The model under review builds one solid part; all positions refer to its coordinate system, in mm. A direction names the side the tool comes from. Coordinates: 2 decimals unless noted, no trailing zeros. Loops run counter-clockwise (first coordinate to the right, second up) from the corner with the lowest first, then second, coordinate; pieces in that order, holes last. Notation, with made-up numbers: (89, -35) - (126, -35) arc R15 ccw to (126, -13) - close; hole circle Ø7 at (-7.75, -11.5). An arc over 180 degrees is marked (long way). Use a Markdown table: item, result. Add a question column.
1) Clearance check with flat-ended pins moving along their axes: pin 1 (1 mm diameter, centred on y = 4, z = 9, fed in from +X); pin 2 (2.5 mm diameter, centred on x = -27.5, z = -22.5, fed in from +Y); pin 3 (3 mm diameter, centred on y = 4.5, z = 17.5, fed in from -X); pin 4 (0.5 mm diameter, centred on x = 27, y = 0.5, fed in from -Z). State where each tip first meets the part, or that it passes through.
2) For faces 4 (the flat face through (26, 1, 21)), 5 (the flat face through (0, 1, 23)), 6 (the flat face through (0, 1, -20)), list the 3-axis set-ups (+Z, -Z, +X, -X, +Y, -Y) from which the entire face can be reached by the end or side of a thin tool; tool diameter is ignored.
3) To check wall thickness, follow L1, parallel to X at y = 0.85, z = 3; L2, parallel to X at y = 0.35, z = 22.5. State the ranges of each line that lie inside material, in increasing order. Write a range as [from, to].
4) Add section C-C, the plane y = 1.7. Give the boundary of the cut face in (x, z).
5) Add section A-A, the plane z = 22.5. Give the boundary of the cut face in (x, y), and give its area (3 significant figures).
6) Add section B-B, the plane x = -27.5. Give the boundary of the cut face in (y, z).
7) Add section D-D, the plane z = -22.5. Give the boundary of the cut face in (x, y).
8) The part is to be moulded in two halves that separate along X. For faces 1 (the flat face through (-3, 2, -25)), 2 (the cylindrical face through (-26.013, 0.507, -22.695)), 3 (the flat face through (15, 1, 20)), say which applies: pulls with the +X half, pulls with the -X half, needs draft (parallel to the pull), parting line crosses it, or undercut.
```python
from build123d import *

# Parameters (mm, degrees)
SKETCH1_W           = 50
SKETCH1_H           = 50
BOSS_EXTRUDE2_DEPTH = 5
SKETCH2_W           = 40
SKETCH2_H           = 40
CUT_EXTRUDE1_DEPTH  = 3
SKETCH3_W           = 5
SKETCH3_H           = 5
BOSS_EXTRUDE3_DEPTH = 1
SKETCH4_R           = 1.5
CUT_EXTRUDE2_DEPTH  = 1
SKETCH6_W           = 10
SKETCH6_H           = 3
CUT_EXTRUDE3_DEPTH  = 10


with BuildPart() as part:
    # Sketch1 → Boss-Extrude2 (new body)
    with BuildSketch(Plane(origin=(0, 0, 0), x_dir=(1, 0, 0), z_dir=(0, 1, 0))):
        Rectangle(SKETCH1_W, SKETCH1_H)
    extrude(amount=BOSS_EXTRUDE2_DEPTH)

    # Sketch2 → Cut-Extrude1 (cut)
    with BuildSketch(Plane(origin=(0, 0, 0), x_dir=(-1, 0, 0), z_dir=(0, -1, 0))):
        Rectangle(SKETCH2_W, SKETCH2_H)
    extrude(amount=-CUT_EXTRUDE1_DEPTH, mode=Mode.SUBTRACT)

    # Sketch3 → Boss-Extrude3 (add)
    with BuildSketch(Plane(origin=(0, 0, 0), x_dir=(-1, 0, 0), z_dir=(0, -1, 0))):
        with Locations((27.5, 22.5)):
            Rectangle(SKETCH3_W, SKETCH3_H)
        with Locations((-27.5, -22.5)):
            Rectangle(SKETCH3_W, SKETCH3_H)
    extrude(amount=-BOSS_EXTRUDE3_DEPTH)

    # Sketch4 → Cut-Extrude2 (cut)
    with BuildSketch(Plane(origin=(0, 1, 0), x_dir=(1, 0, 0), z_dir=(0, 1, 0))):
        with Locations(Location((-27.5, 22.5, 0), (0, 0, 270))):  # turned: the seam where the file's is
            Circle(SKETCH4_R)
        with Locations(Location((27.5, -22.5, 0), (0, 0, 270))):  # turned: the seam where the file's is
            Circle(SKETCH4_R)
    extrude(amount=-CUT_EXTRUDE2_DEPTH, mode=Mode.SUBTRACT)

    # Sketch6 → Cut-Extrude3 (cut)
    with BuildSketch(Plane.XY.offset(25)):
        with Locations((5, 1.5)):
            Rectangle(SKETCH6_W, SKETCH6_H)
    extrude(amount=-CUT_EXTRUDE3_DEPTH, mode=Mode.SUBTRACT)


solid = part.part
```
From the geometry:
| question | item | result |
|---|---|---|
| 1 | pin 1 | stops at x = 25 |
| 1 | pin 2 | passes through |
| 1 | pin 3 | stops at x = -25 |
| 1 | pin 4 | stops at z = 20 |
| 2 | face 4 | +Z, -Z, +X, +Y |
| 2 | face 5 | +Z, -Y |
| 2 | face 6 | -Y |
| 3 | L1 | x = [-25, -20], [20, 25] |
| 3 | L2 | x = [-25, 0], [10, 26], [29, 30] |
| 4 | outline | (-25, -25) - (25, -25) - (25, 25) - (10, 25) - (10, 20) - (20, 20) - (20, -20) - (-20, -20) - (-20, 20) - (0, 20) - (0, 25) - (-25, 25) - close |
| 5 | outline | (-25, 0) - (0, 0) - (0, 3) - (10, 3) - (10, 0) - (26, 0) - (26, 1) - (25, 1) - (25, 5) - (-25, 5) - close; (29, 0) - (30, 0) - (30, 1) - (29, 1) - close |
| 5 | area | 222 mm^2 |
| 6 | outline | (0, -25) - (1, -25) - (1, -24) - (0, -24) - close; (0, -21) - (1, -21) - (1, -20) - (0, -20) - close |
| 7 | outline | (-30, 0) - (-29, 0) - (-29, 1) - (-30, 1) - close; (-26, 0) - (25, 0) - (25, 5) - (-25, 5) - (-25, 1) - (-26, 1) - close |
| 8 | face 1 | needs draft |
| 8 | face 2 | undercut |
| 8 | face 3 | undercut |
